from build123d import *

# Parameters (mm, degrees)
F1_DEPTH = 127
F2_DEPTH = 203.2
F0_R     = 101.6
F0_R_2   = 152.4
F3_DEPTH = 254


with BuildPart() as f1:
    # F0 (on Front) → F1 (new body)
    with BuildSketch(Plane.XZ):
        with BuildLine():
            ThreePointArc((223.864395, -374.003052), (-217.941248, -384.451571), (0, 0))
            Line((0, 0), (-1278.093423, 0))
            ThreePointArc((-1278.093423, 0), (-1098.488301, -74.394878), (-1024.093423, -254))
            ThreePointArc((-1024.093423, -254), (-1287.566511, -507.823286), (-1531.386814, -235.067006))
            ThreePointArc((-1531.386814, -235.067006), (-1461.371729, -848.834442), (-1170.661517, -1393.903384))
            ThreePointArc((-1170.661517, -1393.903384), (-1139.903384, -1108.186011), (-854.186011, -1138.944144))
            ThreePointArc((-854.186011, -1138.944144), (-417.434031, -1483.085525), (125.5956, -1602.686539))
            ThreePointArc((125.5956, -1602.686539), (221.360668, -1625.748682), (295.027596, -1691.139771))
            ThreePointArc((295.027596, -1691.139771), (75.035952, -1042.534849), (223.864395, -374.003052))
        make_face()
    extrude(amount=F1_DEPTH)

    # F0 (on Front) → F2 (join)
    with BuildSketch(Plane.XZ):
        with BuildLine():
            ThreePointArc((129.048784, -2009.071868), (307.452714, -1899.91768), (295.027596, -1691.139771))
            ThreePointArc((295.027596, -1691.139771), (221.360668, -1625.748682), (125.5956, -1602.686539))
            ThreePointArc((125.5956, -1602.686539), (-417.434031, -1483.085525), (-854.186011, -1138.944144))
            ThreePointArc((-854.186011, -1138.944144), (-1139.903384, -1108.186011), (-1170.661517, -1393.903384))
            ThreePointArc((-1170.661517, -1393.903384), (-591.296645, -1850.417461), (129.048784, -2009.071868))
        make_face()
        with BuildLine():
            ThreePointArc((126.458896, -1704.282872), (228.918524, -1805.015908), (128.185488, -1907.475536))
            ThreePointArc((128.185488, -1907.475536), (-547.830991, -1758.584477), (-1091.54264, -1330.163574))
            ThreePointArc((-1091.54264, -1330.163574), (-1076.163574, -1187.304888), (-933.304888, -1202.683954))
            ThreePointArc((-933.304888, -1202.683954), (-460.899684, -1574.918509), (126.458896, -1704.282872))
        make_face(mode=Mode.SUBTRACT)
    extrude(amount=F2_DEPTH)

    # F0 (on Front) → F3 (join)
    with BuildSketch(Plane.XZ):
        with BuildLine():
            ThreePointArc((-1024.093423, -254), (-1098.488301, -74.394878), (-1278.093423, 0))
            ThreePointArc((-1278.093423, 0), (-1450.875106, -67.821348), (-1531.386814, -235.067006))
            ThreePointArc((-1531.386814, -235.067006), (-1287.566511, -507.823286), (-1024.093423, -254))
        make_face()
        with Locations((-1278.093423, -254)):
            Circle(F0_R, mode=Mode.SUBTRACT)
        with BuildLine():
            ThreePointArc((254, -254), (179.605122, -74.394878), (0, 0))
            ThreePointArc((0, 0), (-217.941248, -384.451571), (223.864395, -374.003052))
            ThreePointArc((223.864395, -374.003052), (246.350925, -315.864544), (254, -254))
        make_face()
        with Locations((0, -254)):
            Circle(F0_R_2, mode=Mode.SUBTRACT)
    extrude(amount=F3_DEPTH)


solid = f1.part
CAD build for the part. Positions are in the model's coordinates, mm. A direction names the side the tool comes from. Round coordinates to 2 decimals unless told otherwise and drop trailing zeros. Loops run counter-clockwise (first coordinate to the right, second up) from the corner with the lowest first, then second, coordinate; pieces in that order, holes last. Notation, with made-up numbers: M 28.5,39.25 L 75.5,39.25 A28 cw 75.5,57.25 Z; hole C -19.75,47.25 d10. An arc over 180 degrees is marked long. One line per question, with ' | ' between items. Start each with the question number.
Item 1: Cut at D-D, the plane z = -183. Write the cut outline in (x, y), plus the area to 3 significant figures.
Item 2: Wall check: line 1 (X direction, y = -87.5, z = -183.5); line 2 (Z direction, x = 127.5, y = -192.5); line 3 (Y direction, x = -629.5, z = -1249.5). Give the ranges that are in metal, low to high.
Item 3: Pin check, flat tips, straight feed: pin 1 Ø3 at (x, y) = (-979.5, -189.5) entering from -Z; pin 2 Ø5 at (y, z) = (-47.5, -1189.5) entering from -X; pin 3 Ø2 at (x, z) = (-1233, -777.5) entering from -Y. Stop position of each tip, or through.
Item 4: Cut at B-B, the plane z = -1232. Write the cut outline in (x, y).
Item 5: Two-plate mould, pull along X, no slides. Class faces 4 (the flat face through (-446, -203.2, -1569)), 5 (the cylindrical face through (75.597, -62.611, -1052.227)), 6 (the cylindrical face through (-538.98, -100.18, -1762.74)): pulls with the +X half, pulls with the -X half, needs draft (parallel to the pull), parting line crosses it, or undercut.
Item 6: Cut at A-A, the plane y = -153. Write the cut outline in (x, z).
Item 7: Cut at C-C, the plane x = -1336. Write the cut outline in (y, z), plus the area to 3 significant figures.
Item 8: Which spindle directions (+Z, -Z, +X, -X, +Y, -Y) get a long thin tool onto all of the face, cutting with end or side? Do faces 1 (the cylindrical face through (228.875, -100.178, -1802.782)), 2 (the flat face through (-633, -127, -834)), 3 (the flat face through (-1282, -254, -363)). Say none if no direction does.
Responses:
1) outline: M -1521.97,-254 L -1350.77,-254 L -1350.77,0 L -1521.97,0 Z; M -1205.42,-254 L -1034.22,-254 L -1034.22,-127 L -243.87,-127 L -243.87,-254 L -134.85,-254 L -134.85,0 L -1205.42,0 Z; M 134.85,-254 L 243.87,-254 L 243.87,0 L 134.85,0 Z | area: 243,000 mm²
2) line 1: x = -1522.11 to -1351.25, -1204.93 to -135.11, 135.11 to 244.02 | line 2: z = -2009.08 to -1907.48, -1704.28 to -1602.68, -473.68 to -337.48, -170.52 to -34.32 | line 3: y = -127 to 0
3) pin 1: stops at z = -1595.51 | pin 2: stops at x = -1312.84 | pin 3: stops at y = -127
4) outline: M -1285.75,-127 L -1212.69,-127 L -1212.69,-203.2 L -1108.01,-203.2 L -1108.01,0 L -1285.75,0 Z; M -909,-203.2 L -771.2,-203.2 L -771.2,-127 L 99.66,-127 L 99.66,0 L -909,0 Z
5) face 4: needs draft | face 5: pulls with the +X half | face 6: undercut
6) outline: M -1531.39,-235.07 A254 ccw long -1024.09,-254 A254 ccw -1278.09,0 A254 ccw Z; M -1170.66,-1393.9 A1651 ccw 129.05,-2009.07 A203.2 ccw 295.03,-1691.14 A203.2 ccw 125.6,-1602.69 A1244.6 cw -854.19,-1138.94 A203.2 ccw Z; M 0,0 A254 ccw long 223.86,-374 A254 ccw 254,-254 A254 ccw Z; hole C -1278.09,-254 d203.2; hole M -1091.54,-1330.16 A1549.4 ccw 128.19,-1907.48 A101.6 ccw 126.46,-1704.28 A1346.2 cw -933.3,-1202.68 A101.6 ccw Z; hole C 0,-254 d304.8
7) outline: M -254,-501.31 L -127,-501.31 L -127,-1145.75 L 0,-1145.75 L 0,-337.48 L -254,-337.48 Z; M -254,-170.52 L 0,-170.52 L 0,-6.69 L -254,-6.69 Z | area: 165,000 mm²
8) face 1: +Y, -Y | face 2: -Y | face 3: +Z, -Z, +X, -X, -Y
